Read the model definition and answer for the solid it produces. Units are mm, in the model's axes. Face numbers are marked on the shaded views. A direction names the side the tool comes from. Coordinates: 2 decimals unless noted, no trailing zeros. Loops run counter-clockwise (first coordinate to the right, second up) from the corner with the lowest first, then second, coordinate; pieces in that order, holes last. Notation, with made-up numbers: (-27, 50) -> (-1, 50) arc R28 cw to (-1, 78) -> close; hole circle Ø2 at (21, 59). An arc over 180 degrees is marked (long way). Answer in a Markdown table with one row per item.
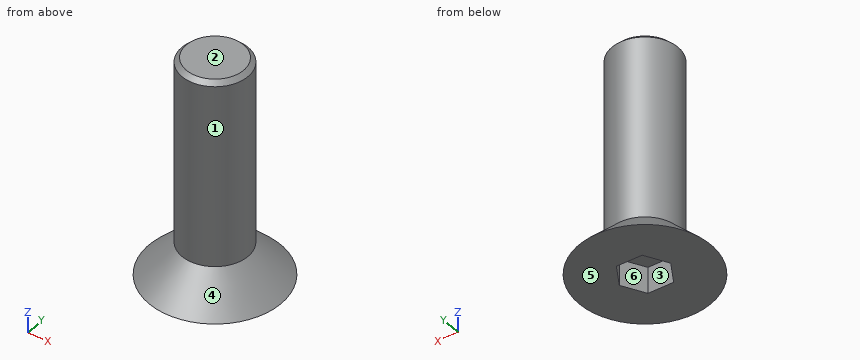
Autodesk Inventor part; units mm, degrees
ref_plane "YZ Plane" through (0, 0, 0) normal (1, 0, 0) x (0, 1, 0)
ref_plane "XZ Plane" through (0, 0, 0) normal (0, 1, 0) x (-1, 0, 0)
ref_plane "XY Plane" through (0, 0, 0) normal (0, 0, 1) x (1, 0, 0)
sketch "Sketch1" plane through (0, 0, 0) normal (1, 0, 0) x (0, 1, 0)
  line L0 (0, 0) -> (0, -10)
  line L1 (0, -10) -> (3, -10)
  line L2 (3, -10) -> (1.5, -8.5)
  line L3 (1.5, -8.5) -> (1.5, 0)
  line L4 (1.5, 0) -> (0, 0)
  dimension "d0" = 6
  dimension "d1" = 10
  dimension "d2" = 45
  dimension "d3" = 3
revolve "Revolution1" add sketch "Sketch1" angle 360 about axis through (0, 0, 0) along (0, 0, -1)
chamfer "Chamfer1" distance 0.2 angle 45 1 edges at (0, -1.5, 0)
thread "Thread1"
sketch "Sketch2" plane through (0, 0, -10) normal (0, 0, -1) x (-1, 0, 0)
  circle A0 centre (0, 0) radius 1.3
  line L0 (1.1547, 0) -> (0.5774, -1)
  line L1 (0.5774, -1) -> (-0.5774, -1)
  line L2 (-0.5774, -1) -> (-1.1547, 0)
  line L3 (-1.1547, 0) -> (-0.5774, 1)
  line L4 (-0.5774, 1) -> (0.5774, 1)
  line L5 (0.5774, 1) -> (1.1547, 0)
  dimension "d10" = 2
extrude "Extrusion1" cut sketch "Sketch2" against normal blind 1.2 contours L0 L1 L2 L3 L4 L5
properties part number "M3 x 10mm FHCS"
1. A cutting plane is placed at A-A on x = 0. Give the vertices of the cut face in (y, z), and give its area (3 significant figures).
A:
| item | result |
|---|---|
| outline | (-3, -10) -> (-1, -10) -> (-1, -8.8) -> (1, -8.8) -> (1, -10) -> (3, -10) -> (1.5, -8.5) -> (1.5, -0.2) -> (1.3, 0) -> (-1.3, 0) -> (-1.5, -0.2) -> (-1.5, -8.5) -> close |
| area | 29.8 mm2 |
2. The mould has two halves that part along X. Classify the marked faces 4, 5 and 6: pulls with the +X half, pulls with the -X half, needs draft (parallel to the pull), parting line crosses it, or undercut.
A:
| item | result |
|---|---|
| face 4 | parting line crosses it |
| face 5 | needs draft |
| face 6 | undercut |
3. A tool of negligible diameter and unlimited length cuts with its end or side. For the marked faces 1, 2 and 3, from which of +Z, -Z, +X, -X, +Y, -Y can it reach the whole face along a straight path? Write none if from no direction.
A:
| item | result |
|---|---|
| face 1 | +Z |
| face 2 | +Z, +X, -X, +Y, -Y |
| face 3 | -Z |
4. Find the intervals of material crossed by probe 1 along Z at (x, y) = (-0.75, 0); probe 2 along Z at (x, y) = (1.5, 0.5); probe 3 along X at (y, z) = (1, -4.75), in increasing order.
A:
| item | result |
|---|---|
| probe 1 | z = -8.8 to 0 |
| probe 2 | z = -10 to -8.58 |
| probe 3 | x = -1.12 to 1.12 |
5. A cutting plane is placed at B-B on z = -7.25. Give the vertices of the cut face in (x, y), and give its area (3 significant figures).
A:
| item | result |
|---|---|
| outline | circle Ø3 at (0, 0) |
| area | 7.07 mm2 |
6. Given pin 1 Ø2 at (x, z) = (0, -2) entering from +Y; pin 2 Ø3 at (x, z) = (2.5, -5.5) entering from +Y; pin 3 Ø0.9 at (x, z) = (0, -9.5) entering from +Y, each flat-ended and moving along its own axis, determine where each tip first touches the part or whether it passes through.
A:
| item | result |
|---|---|
| pin 1 | stops at y = 1.5 |
| pin 2 | stops at y = 1.12 |
| pin 3 | stops at y = 2.95 |
